Build history of the part. All positions in model axes, mm. A direction names the side the tool comes from. Round coordinates to 2 decimals unless told otherwise and drop trailing zeros. Loops run counter-clockwise (first coordinate to the right, second up) from the corner with the lowest first, then second, coordinate; pieces in that order, holes last. Notation, with made-up numbers: (50.25, 27.5) - (74.25, 27.5) arc R19 ccw to (74.25, 33.5) - close; hole circle Ø11 at (81.5, 2.5). An arc over 180 degrees is marked (long way). Use a Markdown table: item, result.
from build123d import *

# Parameters (mm, degrees)
SKETCH1_W           = 69.85
SKETCH1_H           = 69.85
BOSS_EXTRUDE1_DEPTH = 69.85
CUT_EXTRUDE2_DEPTH  = 100
SKETCH3_W           = 69.85
SKETCH3_H           = 6.35
CUT_EXTRUDE4_DEPTH  = 3.81
SKETCH4_W           = 79.375
SKETCH4_H           = 25.4
CUT_EXTRUDE5_DEPTH  = 1.6
SKETCH5_W           = 50
SKETCH5_H           = 21.59
CUT_EXTRUDE6_DEPTH  = 10


with BuildPart() as part:
    # Sketch1 → Boss-Extrude1 (new body)
    with BuildSketch(Plane(origin=(0, 0, 0), x_dir=(1, 0, 0), z_dir=(0, 1, 0))):
        with Locations((34.925, 34.925)):
            Rectangle(SKETCH1_W, SKETCH1_H)
    extrude(amount=BOSS_EXTRUDE1_DEPTH)

    # Sketch2 → Cut-Extrude2 (cut)
    with BuildSketch(Plane(origin=(0, 0, 0), x_dir=(0.707106781, 0, -0.707106781), z_dir=(0.707106781, 0, 0.707106781))):
        Polygon((98.782817332, 69.85), (98.782817332, 0), (49.391408666, 0), (0, 0), (0, 69.85), (49.391408666, 69.85), align=None)
    extrude(amount=CUT_EXTRUDE2_DEPTH, mode=Mode.SUBTRACT)

    # Sketch3 → Cut-Extrude4 (cut)
    with BuildSketch(Plane(origin=(0, 0, 0), x_dir=(0.707106781, 0, -0.707106781), z_dir=(0.707106781, 0, 0.707106781))):
        with Locations((49.391408666, 5.715)):
            Rectangle(SKETCH3_W, SKETCH3_H)
        with Locations((49.391408666, 64.135)):
            Rectangle(SKETCH3_W, SKETCH3_H)
    extrude(amount=-CUT_EXTRUDE4_DEPTH, mode=Mode.SUBTRACT)

    # Sketch4 → Cut-Extrude5 (cut)
    with BuildSketch(Plane(origin=(0, 0, 0), x_dir=(0.707106781, 0, -0.707106781), z_dir=(0.707106781, 0, 0.707106781))):
        with Locations((49.391408666, 34.925)):
            Rectangle(SKETCH4_W, SKETCH4_H)
    extrude(amount=-CUT_EXTRUDE5_DEPTH, mode=Mode.SUBTRACT)

    # Sketch5 → Cut-Extrude6 (cut)
    with BuildSketch(Plane(origin=(-1.13137085, 0, -1.13137085), x_dir=(0.707106781, 0, -0.707106781), z_dir=(0.707106781, 0, 0.707106781))):
        with Locations((49.391408666, 34.925)):
            Rectangle(SKETCH5_W, SKETCH5_H)
    extrude(amount=-CUT_EXTRUDE6_DEPTH, mode=Mode.SUBTRACT)


solid = part.part
Q1. Probe line 1 (Y direction, x = 47, z = -52); line 2 (Y direction, x = 36, z = -49); line 3 (X direction, y = 58.5, z = -47). List the from-to ranges inside material, lowest first.
Results found:
| item | result |
|---|---|
| line 1 | y = 0 to 2.54, 8.89 to 24.13, 45.72 to 60.96, 67.31 to 69.85 |
| line 2 | y = 0 to 24.13, 45.72 to 69.85 |
| line 3 | x = 0 to 47 |
Q2. Which spindle directions (+Z, -Z, +X, -X, +Y, -Y) get a long thin tool onto all of the face, cutting with end or side? Do faces 5 (the face through (58.29, 5.67, -60.95)), 6 (the face through (27, 0, -43)). Say none if no direction does.
Results found:
| item | result |
|---|---|
| face 5 | +Z |
| face 6 | +Z, -Z, +X, -X, -Y |
Q3. Cut at A-A, the plane y = 35.5. List the corners of the cut face in (x, z).
Results found:
| item | result |
|---|---|
| outline | (0, -69.85) - (69.85, -69.85) - (62.99, -62.99) - (61.86, -64.12) - (51.47, -53.73) - (44.4, -60.81) - (9.04, -25.45) - (16.12, -18.38) - (5.73, -7.99) - (6.86, -6.86) - (0, 0) - close |
Q4. Drop flat-ended pins along their axis: pin 1 (8 mm diameter, centred on x = 12, y = 9.5, fed in from +Z); pin 2 (8 mm diameter, centred on y = 8, z = -33.5, fed in from +X); pin 3 (6 mm diameter, centred on y = 30.5, z = -25.5, fed in from -X); pin 4 (8 mm diameter, centred on y = 28.5, z = -23, fed in from +X). Give the stop position or say it passes through.
Results found:
| item | result |
|---|---|
| pin 1 | stops at z = -8 |
| pin 2 | stops at x = 37.4 |
| pin 3 | stops at x = 0 |
| pin 4 | stops at x = 15.49 |
Q5. Cut at D-D, the plane z = -21. List the corners of the cut face in (x, y) (3 decimals).
Results found:
| item | result |
|---|---|
| outline | (0, 0) - (21, 0) - (21, 2.54) - (15.612, 2.54) - (15.612, 8.89) - (21, 8.89) - (21, 22.225) - (18.737, 22.225) - (18.737, 24.13) - (13.495, 24.13) - (13.495, 45.72) - (18.737, 45.72) - (18.737, 47.625) - (21, 47.625) - (21, 60.96) - (15.612, 60.96) - (15.612, 67.31) - (21, 67.31) - (21, 69.85) - (0, 69.85) - close |
Q6. Pull direction Z, two halves, no side cores. Call faces 1 (the face through (35, 51, -35)), 2 (the face through (26.475, 35.076, -42.88)), 3 (the face through (8.9, 5.67, -11.56)), 4 (the face through (27, 69.85, -43)): pulls with the +Z half, pulls with the -Z half, needs draft (parallel to the pull), parting line crosses it, or undercut.
Results found:
| item | result |
|---|---|
| face 1 | pulls with the +Z half |
| face 2 | undercut |
| face 3 | undercut |
| face 4 | needs draft |
Q7. Cut at B-B, the plane x = 55. List the corners of the cut face in (y, z) (3 decimals).
Results found:
| item | result |
|---|---|
| outline | (0, -69.85) - (69.85, -69.85) - (69.85, -55) - (67.31, -55) - (67.31, -60.388) - (60.96, -60.388) - (60.96, -55) - (47.625, -55) - (47.625, -57.263) - (22.225, -57.263) - (22.225, -55) - (8.89, -55) - (8.89, -60.388) - (2.54, -60.388) - (2.54, -55) - (0, -55) - close |
Q8. Cut at C-C, the plane z = -57.5. List the corners of the cut face in (x, y) (3 decimals), plus the area to 3 significant figures.
Results found:
| item | result |
|---|---|
| outline | (0, 0) - (57.5, 0) - (57.5, 2.54) - (52.112, 2.54) - (52.112, 8.89) - (57.5, 8.89) - (57.5, 22.225) - (55.237, 22.225) - (55.237, 47.625) - (57.5, 47.625) - (57.5, 60.96) - (52.112, 60.96) - (52.112, 67.31) - (57.5, 67.31) - (57.5, 69.85) - (0, 69.85) - close; hole (41.095, 24.13) - (47.705, 24.13) - (47.705, 45.72) - (41.095, 45.72) - close |
| area | 3,750 mm2 |
